Autodesk Inventor part; units mm, degrees
ref_plane "YZ Plane" through (0, 0, 0) normal (1, 0, 0) x (0, 1, 0)
ref_plane "XZ Plane" through (0, 0, 0) normal (0, 1, 0) x (-1, 0, 0)
ref_plane "XY Plane" through (0, 0, 0) normal (0, 0, 1) x (1, 0, 0)
sketch "Sketch1" plane through (0, 0, 0) normal (0, 0, 1) x (1, 0, 0)
  circle A0 centre (0, 0) radius 25.6
  circle A1 centre (0, 44.45) radius 3.3734
  circle A2 centre (-38.4948, 22.225) radius 3.3734
  circle A3 centre (-38.4948, -22.225) radius 3.3734
  circle A4 centre (0, -44.45) radius 3.3734
  circle A5 centre (38.4948, -22.225) radius 3.3734
  circle A6 centre (38.4948, 22.225) radius 3.3734
  circle A7 centre (0, 0) radius 57.15
  dimension "d0" = 51.2
  dimension "d1" = 44.45
  dimension "d2" = 6.7469
  dimension "d5" = 360
  dimension "d7" = 114.3
extrude "Extrusion1" add sketch "Sketch1" along normal blind 25.4
properties part number "IndexerWheelSpacer"
Can you work these out from the model? Positions are in its coordinate system, mm. Give positions to 0.01 mm unless a question says otherwise; leave off trailing zeros. Order: outer loops, then holes, each group sorted by start corner. A loop starts at its lowest first (then second) coordinate and runs counter-clockwise, first axis right, second up. Notation, with made-up numbers: M -28,74.25 L 18,74.25 A21 ccw 18,87.25 Z; hole C 53.25,76 d1. An arc over 180 degrees is marked long. Use one line per item in the form item = value. Start each with the question number.
Item 1: If we section it at B-B (y = -9): Write out the boundary of the cut face in (x, z), then the cut area to 3 significant figures.
Item 2: If we section it at D-D (x = 23.5): Write out the boundary of the cut face in (y, z), then the cut area to 3 significant figures.
Item 3: If we section it at A-A (x = 0): Write out the boundary of the cut face in (y, z), then the cut area to 3 significant figures.
Item 4: If we section it at C-C (z = 2.5): Write out the boundary of the cut face in (x, y) (3 decimals).
Item 5: We'd pull the mould along Y, two halves only. Please class faces 1 (the cylindrical face through (-20.3, 15.6, 12.5)), 2 (the flat face through (-1, 26, 25.4)), 3 (the cylindrical face through (-57.095, -2.513, 12.522)): +Y half, -Y half, draft (parallel to the pull), parting line (faces both ways), or undercut.
Item 6: Will these pins go through, and if not, where does the flat tip stop? pin 1 Ø1 at (y, z) = (-12.5, 11.5) entering from +X; pin 2 Ø6 at (x, y) = (44.5, 40) entering from -Z; pin 3 Ø4 at (y, z) = (26, 6.5) entering from -X; pin 4 Ø3 at (y, z) = (43.5, 14.5) entering from -X.
Item 7: If I drill on line 1 along Y through (x, z) = (0, 12.5); line 2 along Y through (x, z) = (-38, 1.5); line 3 along Y through (x, z) = (-36.5, 23), over which ranges is the centre line in solid material (lowest first)?
Outcome:
q1.outline = M -56.44,0 L -23.97,0 L -23.97,25.4 L -56.44,25.4 Z; M 23.97,0 L 56.44,0 L 56.44,25.4 L 23.97,25.4 Z
q1.area = 1,650 mm2
q2.outline = M -52.09,0 L -10.15,0 L -10.15,25.4 L -52.09,25.4 Z; M 10.15,0 L 52.09,0 L 52.09,25.4 L 10.15,25.4 Z
q2.area = 2,130 mm2
q3.outline = M -57.15,0 L -47.82,0 L -47.82,25.4 L -57.15,25.4 Z; M -41.08,0 L -25.6,0 L -25.6,25.4 L -41.08,25.4 Z; M 25.6,0 L 41.08,0 L 41.08,25.4 L 25.6,25.4 Z; M 47.82,0 L 57.15,0 L 57.15,25.4 L 47.82,25.4 Z
q3.area = 1,260 mm2
q4.outline = C 0,0 d114.3; hole C -38.495,-22.225 d6.747; hole C -38.495,22.225 d6.747; hole C 0,0 d51.2; hole C 0,-44.45 d6.747; hole C 0,44.45 d6.747; hole C 38.495,-22.225 d6.747; hole C 38.495,22.225 d6.747
q5.face_1 = undercut
q5.face_2 = draft
q5.face_3 = parting line
q6.pin_1 = 55.88
q6.pin_2 = 0
q6.pin_3 = -51.87
q6.pin_4 = -38.76
q7.line_1 = -57.15 to -47.82, -41.08 to -25.6, 25.6 to 41.08, 47.82 to 57.15
q7.line_2 = -42.69 to -25.56, -18.89 to 18.89, 25.56 to 42.69
q7.line_3 = -43.98 to -24.95, -19.5 to 19.5, 24.95 to 43.98
